Part model, mm, in its own coordinate system. A direction names the side the tool comes from. Round coordinates to 2 decimals unless told otherwise and drop trailing zeros. Loops run counter-clockwise (first coordinate to the right, second up) from the corner with the lowest first, then second, coordinate; pieces in that order, holes last. Notation, with made-up numbers: (38.25, 13.5) -> (95.25, 13.5) arc R25 cw to (95.25, 52.5) -> close; hole circle Ø1 at (-17.75, 83.25). An arc over 180 degrees is marked (long way). Use a Markdown table: item, result. Add a question column.
Item 1: Flat gauge pins, fed straight in: pin 1 (6 mm diameter, centred on y = -8, z = 6.5, fed in from +X); pin 2 (5.5 mm diameter, centred on y = -10, z = 6.622, fed in from -X); pin 3 (4 mm diameter, centred on y = -16, z = -6, fed in from -X); pin 4 (1.6 mm diameter, centred on y = -10.5, z = 6, fed in from -X). Where does each tip first touch, or does it go through?
Item 2: Two-plate mould, pull along Z, no slides. Class faces 5 (the face through (-6.94, -9.86, -7.28)), 6 (the face through (-4.046, -3.313, 6.397)), 7 (the face through (-3, -11, 5)), 8 (the face through (4, 0, -4)): pulls with the +Z half, pulls with the -Z half, needs draft (parallel to the pull), parting line crosses it, or undercut.
Item 3: Cut at A-A, the plane x = 3. List the corners of the cut face in (y, z), plus the area to 3 significant figures.
Item 4: Cut at D-D, the plane x = 0. List the corners of the cut face in (y, z), plus the area to 3 significant figures.
Item 5: Cut at C-C, the plane z = 2. List the corners of the cut face in (x, y).
Item 6: Which spindle directions (+Z, -Z, +X, -X, +Y, -Y) get a long thin tool onto all of the face, cutting with end or side? Do faces 1 (the face through (1.789, -9.9, 4.7)), 2 (the face through (6.95, -9.86, -7.23)), 3 (the face through (-7, -10, -10)), 4 (the face through (3.789, -9.9, 8.5)). Say none if no direction does.
Item 7: Probe line 1 (X direction, y = -6.75, z = -9); line 2 (Z direction, x = 2.65, y = -10); line 3 (X direction, y = -12.5, z = -5). List the from-to ranges inside material, lowest first. Write a range as [from, to].
Item 8: Cut at B-B, the plane z = -9. List the corners of the cut face in (x, y).
```python
from build123d import *

# Parameters (mm, degrees)
F1_DEPTH     = 20
F2_R         = 3.5
F2_R_2       = 1.7
F3_DEPTH     = 4
F4_DEPTH     = 25
F5_T1_DEPTH  = 20
F5_T6_DEPTH  = 12.1022846539
F5_S7_R      = 1.7
F5_T8_DEPTH  = 8
F5_T12_DEPTH = 12.1022846539
F5_S13_R     = 1.7
F5_T14_DEPTH = 8
F5_T18_DEPTH = 10.2630041323
F5_S19_R     = 3.5
F5_T20_DEPTH = 7
F5_T24_DEPTH = 10.2630041323
F5_S25_R     = 3.5
F5_T26_DEPTH = 7
F5_T27_DEPTH = 23.3663915102
F5_T29_DEPTH = 22.9020360067
F6_R         = 3.5
F6_R_2       = 1.7
F7_DEPTH     = 12
F8_DEPTH     = 12
F9_DEPTH     = 6
F10_DEPTH    = 10


# Not quite as in the source:
# - a fillet or chamfer that OpenCascade refuses, or shapes differently, is made with other operations: its cross-section is extruded or revolved along the edge and cut away or added


with BuildPart() as f1:
    # F0 (on Front) → F1 (new body)
    with BuildSketch(Plane.XZ):
        with BuildLine():
            ThreePointArc((-1.7, -3.8405728739), (-4.1997120304, -0.0491819207), (-1.7894736842, 3.7997084011))
            Line((-1.7894736842, 3.7997084011), (-1.7894736842, 9.1220820965))
            Line((-1.7894736842, 9.1220820965), (-3.7894736842, 9.1220820965))
            Line((-3.7894736842, 9.1220820965), (-3.7894736842, 6.1220820965))
            ThreePointArc((-3.7894736842, 6.1220820965), (-6.8557776995, 2.199616361), (-6.6439040907, -2.7746240166))
            add(Edge.make_bspline(
                [(-6.6356726702, -2.7942527112), (-6.6390399212, -2.7803089062), (-6.6413283577, -2.7774058988), (-6.6439040907, -2.7746240166)],
                knots=[0.9532514843, 0.9532514843, 0.9532514843, 0.9532514843, 1, 1, 1, 1], degree=3))
            add(Edge.make_bspline(
                [(-7, -7.2), (-6.7795680226, -6.7700727801), (-6.2785456929, -5.7974600377), (-6.5973790049, -2.9528269921), (-6.6356726702, -2.7942527112)],
                knots=[0, 0, 0, 0, 0.4216094964, 0.9532514843, 0.9532514843, 0.9532514843, 0.9532514843], degree=3))
            Line((-7, -7.2), (-7, -13.2))
            Line((-7, -13.2), (-1.7, -13.2))
            Line((-1.7, -13.2), (-1.7, -4.2))
            Line((-1.7, -4.2), (-1.7, -3.8405728739))
        make_face()
        with BuildLine():
            ThreePointArc((1.7, -3.8405728739), (0, -4.2), (-1.7, -3.8405728739))
            Line((-1.7, -3.8405728739), (-1.7, -4.2))
            Line((-1.7, -4.2), (-1.7, -13.2))
            Line((-1.7, -13.2), (1.7, -13.2))
            Line((1.7, -13.2), (1.7, -4.2))
            Line((1.7, -4.2), (1.7, -3.8405728739))
        make_face()
        with BuildLine():
            ThreePointArc((1.7894736842, 3.7997084011), (4.1997120304, -0.0491819207), (1.7, -3.8405728739))
            Line((1.7, -3.8405728739), (1.7, -4.2))
            Line((1.7, -4.2), (1.7, -13.2))
            Line((1.7, -13.2), (7, -13.2))
            Line((7, -13.2), (7, -7.2))
            add(Edge.make_bspline(
                [(7, -7.2), (6.7871491537, -6.6864508711), (6.3058923114, -5.5253136877), (6.5175995563, -3.7720698099), (6.6356726702, -2.7942527112)],
                knots=[0, 0, 0, 0, 0.4422811845, 1, 1, 1, 1], degree=3))
            ThreePointArc((6.6356726702, -2.7942527112), (6.8590214848, 2.1894803656), (3.7894736842, 6.1220820965))
            Line((3.7894736842, 6.1220820965), (3.7894736842, 9.1220820965))
            Line((3.7894736842, 9.1220820965), (1.7894736842, 9.1220820965))
            Line((1.7894736842, 9.1220820965), (1.7894736842, 3.7997084011))
        make_face()
        with BuildLine():
            add(Edge.make_bspline(
                [(-6.6356726702, -2.7942527112), (-6.6390399212, -2.7803089062), (-6.6413283577, -2.7774058988), (-6.6439040907, -2.7746240166)],
                knots=[0.9532514843, 0.9532514843, 0.9532514843, 0.9532514843, 1, 1, 1, 1], degree=3))
            ThreePointArc((-6.6439040907, -2.7746240166), (-6.6397956338, -2.7844414056), (-6.6356726702, -2.7942527112))
        make_face()
    extrude(amount=F1_DEPTH)

    # F2 (on face) → F3 (cut)
    with BuildSketch(Plane(origin=(-7, 0, 0), x_dir=(0, -1, 0), z_dir=(-1, 0, 0))):
        with Locations((10, 6.622)):
            Circle(F2_R)
        with Locations((10, 6.622)):
            Circle(F2_R_2, mode=Mode.SUBTRACT)
    extrude(amount=-F3_DEPTH, mode=Mode.SUBTRACT)

    # F2 (on face) → F4 (cut)
    with BuildSketch(Plane(origin=(-7, 0, 0), x_dir=(0, -1, 0), z_dir=(-1, 0, 0))):
        with Locations((10, 6.622)):
            Circle(F2_R_2)
    extrude(amount=-F4_DEPTH, mode=Mode.SUBTRACT)

    # F5: fillet of radius 3 on 8 edges, made by hand

    # F5_s2 → F5_t1 (join)
    with BuildSketch(Plane.XZ):
        with BuildLine():
            ThreePointArc((-6.7483493849, -2.5087886996), (-6.6395606645, -2.8691274316), (-6.5767127025, -3.2402461743))
            Line((-6.5767127025, -3.2402461743), (-6.2781272304, -3.2087696206))
            ThreePointArc((-6.2781272304, -3.2087696206), (-6.304537605, -2.9799785061), (-6.343821894, -2.723774473))
            Line((-6.343821894, -2.723774473), (-6.3589651198, -2.6777323732))
            ThreePointArc((-6.3589651198, -2.6777323732), (-6.4145893512, -2.5416001874), (-6.466927581, -2.4041663985))
            Line((-6.466927581, -2.4041663985), (-6.7483493849, -2.5087886996))
        make_face()
        with BuildLine():
            ThreePointArc((6.5887317904, -3.1834061265), (6.6509501418, -2.8334452349), (6.754091056, -2.4932898281))
            Line((6.754091056, -2.4932898281), (6.4724298111, -2.3893138658))
            ThreePointArc((6.4724298111, -2.3893138658), (6.4175024363, -2.534235691), (6.3589651198, -2.6777323732))
            Line((6.3589651198, -2.6777323732), (6.3375979172, -2.7582596669))
            ThreePointArc((6.3375979172, -2.7582596669), (6.3141276632, -2.9530960278), (6.290534619, -3.1484417941))
            Line((6.290534619, -3.1484417941), (6.5887317904, -3.1834061265))
        make_face()
    extrude(amount=F5_T1_DEPTH)


with BuildPart() as f5_tool4:
    # F5_s5 → F5_t6 (new body)
    with BuildSketch(Plane.XZ.offset(7.8977153461)):
        with BuildLine():
            ThreePointArc((4.792775332, 5.3724803189), (4.0514647707, 6.385428811), (3.7890736842, 7.6129290813))
            Line((3.7890736842, 7.6129290813), (3.4888336842, 7.6129290813))
            ThreePointArc((3.4888336842, 7.6129290813), (3.4892336842, 6.8675055889), (3.4892336842, 6.1220820965))
            Line((3.4892336842, 6.1220820965), (3.6314526316, 5.8667912731))
            ThreePointArc((3.6314526316, 5.8667912731), (4.1279416848, 5.5287236777), (4.5929054968, 5.1484354427))
            Line((4.5929054968, 5.1484354427), (4.792775332, 5.3724803189))
        make_face()
    extrude(amount=F5_T6_DEPTH)

    # F5_s7 → F5_t8 (cut, symmetric)
    with BuildSketch(Plane.YZ.offset(4.1)):
        with Locations((-10, 6.622)):
            Circle(F5_S7_R)
    extrude(amount=F5_T8_DEPTH, both=True, mode=Mode.SUBTRACT)


with BuildPart() as f1_1:
    add(f1.part)

    # F5_t3: union F5_tool4
    add(f5_tool4.part)


with BuildPart() as f5_tool10:
    # F5_s11 → F5_t12 (new body)
    with BuildSketch(Plane.XZ):
        with BuildLine():
            ThreePointArc((4.792775332, 5.3724803189), (4.0514647707, 6.385428811), (3.7890736842, 7.6129290813))
            Line((3.7890736842, 7.6129290813), (3.4888336842, 7.6129290813))
            ThreePointArc((3.4888336842, 7.6129290813), (3.4892336842, 6.8675055889), (3.4892336842, 6.1220820965))
            Line((3.4892336842, 6.1220820965), (3.6314526316, 5.8667912731))
            ThreePointArc((3.6314526316, 5.8667912731), (4.1279416848, 5.5287236777), (4.5929054968, 5.1484354427))
            Line((4.5929054968, 5.1484354427), (4.792775332, 5.3724803189))
        make_face()
    extrude(amount=F5_T12_DEPTH)

    # F5_s13 → F5_t14 (cut, symmetric)
    with BuildSketch(Plane.YZ.offset(4.1)):
        with Locations((-10, 6.622)):
            Circle(F5_S13_R)
    extrude(amount=F5_T14_DEPTH, both=True, mode=Mode.SUBTRACT)


with BuildPart() as f1_2:
    add(f1_1.part)

    # F5_t9: union F5_tool10
    add(f5_tool10.part)


with BuildPart() as f5_tool16:
    # F5_s17 → F5_t18 (new body)
    with BuildSketch(Plane.XZ):
        with BuildLine():
            ThreePointArc((-3.7890736842, 7.6129290813), (-4.0514647707, 6.385428811), (-4.792775332, 5.3724803189))
            Line((-4.792775332, 5.3724803189), (-4.5929054968, 5.1484354427))
            ThreePointArc((-4.5929054968, 5.1484354427), (-4.1279416848, 5.5287236777), (-3.6314526316, 5.8667912731))
            Line((-3.6314526316, 5.8667912731), (-3.4892336842, 6.1220820965))
            ThreePointArc((-3.4892336842, 6.1220820965), (-3.4892336842, 6.8675055889), (-3.4888336842, 7.6129290813))
            Line((-3.4888336842, 7.6129290813), (-3.7890736842, 7.6129290813))
        make_face()
    extrude(amount=F5_T18_DEPTH)

    # F5_s19 → F5_t20 (cut, symmetric)
    with BuildSketch(Plane.YZ.offset(-4.1)):
        with Locations((-10, 6.622)):
            Circle(F5_S19_R)
    extrude(amount=F5_T20_DEPTH, both=True, mode=Mode.SUBTRACT)


with BuildPart() as f1_3:
    add(f1_2.part)

    # F5_t15: union F5_tool16
    add(f5_tool16.part)


with BuildPart() as f5_tool22:
    # F5_s23 → F5_t24 (new body)
    with BuildSketch(Plane.XZ.offset(9.7369958677)):
        with BuildLine():
            ThreePointArc((-4.792775332, 5.3724803189), (-4.0514647707, 6.385428811), (-3.7890736842, 7.6129290813))
            Line((-3.7890736842, 7.6129290813), (-3.4888336842, 7.6129290813))
            ThreePointArc((-3.4888336842, 7.6129290813), (-3.4892336842, 6.8675055889), (-3.4892336842, 6.1220820965))
            Line((-3.4892336842, 6.1220820965), (-3.6314526316, 5.8667912731))
            ThreePointArc((-3.6314526316, 5.8667912731), (-4.1279416848, 5.5287236777), (-4.5929054968, 5.1484354427))
            Line((-4.5929054968, 5.1484354427), (-4.792775332, 5.3724803189))
        make_face()
    extrude(amount=F5_T24_DEPTH)

    # F5_s25 → F5_t26 (cut, symmetric)
    with BuildSketch(Plane.YZ.offset(-4.1)):
        with Locations((-10, 6.622)):
            Circle(F5_S25_R)
    extrude(amount=F5_T26_DEPTH, both=True, mode=Mode.SUBTRACT)


with BuildPart() as f1_4:
    add(f1_3.part)

    # F5_t21: union F5_tool22
    add(f5_tool22.part)

    # F5_s28 → F5_t27 (cut)
    with BuildSketch(Plane.XZ.offset(-1.6831957551)):
        with BuildLine():
            ThreePointArc((-7.0004, -7.8732781832), (-6.9416848839, -7.2824101234), (-6.7678360085, -6.7146521667))
            Line((-6.7678360085, -6.7146521667), (-7.0448196093, -6.5987895651))
            ThreePointArc((-7.0448196093, -6.5987895651), (-7.148871707, -6.8283644641), (-7.2671697753, -7.0630169034))
            Line((-7.2671697753, -7.0630169034), (-7.30024, -7.2))
            ThreePointArc((-7.30024, -7.2), (-7.30024, -7.5366390916), (-7.30064, -7.8732781832))
            Line((-7.30064, -7.8732781832), (-7.0004, -7.8732781832))
        make_face()
    extrude(amount=F5_T27_DEPTH, mode=Mode.SUBTRACT)

    # F5_s30 → F5_t29 (cut)
    with BuildSketch(Plane.XZ.offset(-1.4510180034)):
        with BuildLine():
            ThreePointArc((6.8044646756, -6.7135604089), (6.9510099307, -7.2380620544), (7.0004, -7.7804070635))
            Line((7.0004, -7.7804070635), (7.30064, -7.7804070635))
            ThreePointArc((7.30064, -7.7804070635), (7.30024, -7.4902035318), (7.30024, -7.2))
            Line((7.30024, -7.2), (7.277360411, -7.0850423555))
            ThreePointArc((7.277360411, -7.0850423555), (7.178454263, -6.8447161783), (7.0851111432, -6.6068757434))
            Line((7.0851111432, -6.6068757434), (6.8044646756, -6.7135604089))
        make_face()
    extrude(amount=F5_T29_DEPTH, mode=Mode.SUBTRACT)

    # F6 (on face) → F7 (cut)
    with BuildSketch(Plane(origin=(0, 0, -13.2), x_dir=(1, 0, 0), z_dir=(0, 0, -1))):
        with Locations((0, 10)):
            Circle(F6_R)
        with Locations((0, 10)):
            Circle(F6_R_2, mode=Mode.SUBTRACT)
    extrude(amount=-F7_DEPTH, mode=Mode.SUBTRACT)

    # F8 (cut): a face of the model
    f8_faces = [f1_4.faces().sort_by_distance(p)[0] for p in [
        (0, -10, -13.2),
    ]]
    extrude(f8_faces, amount=-F8_DEPTH, mode=Mode.SUBTRACT)

    # F6 (on face) → F9 (join)
    with BuildSketch(Plane(origin=(0, 0, -13.2), x_dir=(1, 0, 0), z_dir=(0, 0, -1))):
        with Locations((0, 10)):
            Circle(F6_R)
        with Locations((0, 10)):
            Circle(F6_R_2, mode=Mode.SUBTRACT)
    extrude(amount=-F9_DEPTH)

    # F0 (on Front) → F10 (cut)
    with BuildSketch(Plane.XZ):
        with BuildLine():
            ThreePointArc((1.7, -3.8405728739), (0, -4.2), (-1.7, -3.8405728739))
            Line((-1.7, -3.8405728739), (-1.7, -4.2))
            Line((-1.7, -4.2), (-1.7, -13.2))
            Line((-1.7, -13.2), (1.7, -13.2))
            Line((1.7, -13.2), (1.7, -4.2))
            Line((1.7, -4.2), (1.7, -3.8405728739))
        make_face()
    extrude(amount=F10_DEPTH, mode=Mode.SUBTRACT)


solid = f1_4.part
```
A:
| question | item | result |
|---|---|---|
| 1 | pin 1 | stops at x = 6.29 |
| 1 | pin 2 | stops at x = -3 |
| 1 | pin 3 | stops at x = -7 |
| 1 | pin 4 | passes through |
| 2 | face 5 | undercut |
| 2 | face 6 | pulls with the +Z half |
| 2 | face 7 | undercut |
| 2 | face 8 | needs draft |
| 3 | outline | (-20, -13.2) -> (0, -13.2) -> (0, -2.94) -> (-8.2, -2.94) -> (-8.2, -7.2) -> (-11.8, -7.2) -> (-11.8, -2.94) -> (-20, -2.94) -> close; (-20, 2.94) -> (0, 2.94) -> (0, 9.12) -> (-20, 9.12) -> close; hole circle Ø3.4 at (-10, 6.62) |
| 3 | area | 304 mm^2 |
| 4 | outline | (-20, -13.2) -> (-11.7, -13.2) -> (-11.7, -7.2) -> (-13.5, -7.2) -> (-13.5, -4.2) -> (-20, -4.2) -> close |
| 4 | area | 69.3 mm^2 |
| 5 | outline | (-6.92, -20) -> (-3.69, -20) -> (-3.69, 0) -> (-6.92, 0) -> close; (3.69, -20) -> (6.92, -20) -> (6.92, 0) -> (3.69, 0) -> close |
| 6 | face 1 | +Z, +Y, -Y |
| 6 | face 2 | +X, +Y, -Y |
| 6 | face 3 | -Z, -X, +Y, -Y |
| 6 | face 4 | +Z, +X, +Y, -Y |
| 7 | line 1 | x = [-7, -1.7], [1.7, 7] |
| 7 | line 2 | z = [-13.2, -7.2], [3.26, 4.92], [8.32, 9.12] |
| 7 | line 3 | x = [-6.48, -2.45], [2.45, 6.46] |
| 8 | outline | (-7, -20) -> (7, -20) -> (7, 0) -> (1.7, 0) -> (1.7, -10) arc R1.7 cw to (-1.7, -10) -> (-1.7, 0) -> (-7, 0) -> close |
